```python
from build123d import *

# Parameters (mm, degrees)
EXTRUDE1_DEPTH = 5


with BuildPart() as part:
    # Sketch1 → Extrude1 (new body)
    with BuildSketch(Plane.XY):
        with BuildLine():
            Line((9.079809995, -4.626394269), (93.079809995, -47.426532026))
            ThreePointArc((93.079809995, -47.426532026), (101.052803287, -54.796691216), (104, -65.24666251))
            Line((104, -65.24666251), (104, -67))
            ThreePointArc((104, -67), (104.878679656, -69.121320344), (107, -70))
            Line((107, -70), (118.700463999, -70))
            ThreePointArc((118.700463999, -70), (120.442572866, -69.442346555), (121.537019726, -67.976704463))
            Line((121.537019726, -67.976704463), (140.410371512, -13.164510908))
            ThreePointArc((140.410371512, -13.164510908), (141.225712031, -9.954099936), (141.5, -6.653147818))
            Line((141.5, -6.653147818), (141.5, 17))
            ThreePointArc((141.5, 17), (140.621320344, 19.121320344), (138.5, 20))
            Line((138.5, 20), (122.5, 20))
            ThreePointArc((122.5, 20), (120.378679656, 19.121320344), (119.5, 17))
            Line((119.5, 17), (119.5, 16.5))
            ThreePointArc((119.5, 16.5), (95.5, -7.5), (71.5, 16.5))
            Line((71.5, 16.5), (71.5, 17))
            ThreePointArc((71.5, 17), (70.621320344, 19.121320344), (68.5, 20))
            Line((68.5, 20), (65, 20))
            ThreePointArc((65, 20), (62.878679656, 20.878679656), (62, 23))
            Line((62, 23), (62, 37))
            ThreePointArc((62, 37), (61.121320344, 39.121320344), (59, 40))
            Line((59, 40), (33.68653561, 40))
            ThreePointArc((33.68653561, 40), (31.795766306, 39.329161102), (30.750598067, 37.616660959))
            add(Edge.make_bspline(
                [(-38.750598067, 37.616660959), (-35.050414777, 20), (-4, 20), (27.050414777, 20), (30.750598067, 37.616660959)],
                knots=[3.261043467, 3.261043467, 3.261043467, 4.71238898, 4.71238898, 6.163734494, 6.163734494, 6.163734494], degree=2, weights=[1, 0.748053124, 1, 0.748053124, 1]))
            ThreePointArc((-38.750598067, 37.616660959), (-39.795766306, 39.329161102), (-41.68653561, 40))
            Line((-41.68653561, 40), (-54.5, 40))
            ThreePointArc((-54.5, 40), (-56.621320344, 39.121320344), (-57.5, 37))
            Line((-57.5, 37), (-57.5, 17.148970879))
            ThreePointArc((-57.5, 17.148970879), (-59.693566818, 5.888319313), (-65.953484912, -3.725599478))
            Line((-65.953484912, -3.725599478), (-87.272335061, -25.73069556))
            ThreePointArc((-87.272335061, -25.73069556), (-88.084372164, -27.372329), (-87.790703125, -29.180124095))
            Line((-87.790703125, -29.180124095), (-82.861971499, -38.853304561))
            ThreePointArc((-82.861971499, -38.853304561), (-81.11600291, -40.344502611), (-78.826980427, -40.164352635))
            Line((-78.826980427, -40.164352635), (-9.079809995, -4.626394269))
            ThreePointArc((-9.079809995, -4.626394269), (0, -2.446524753), (9.079809995, -4.626394269))
        make_face()
    extrude(amount=EXTRUDE1_DEPTH)


solid = part.part
```
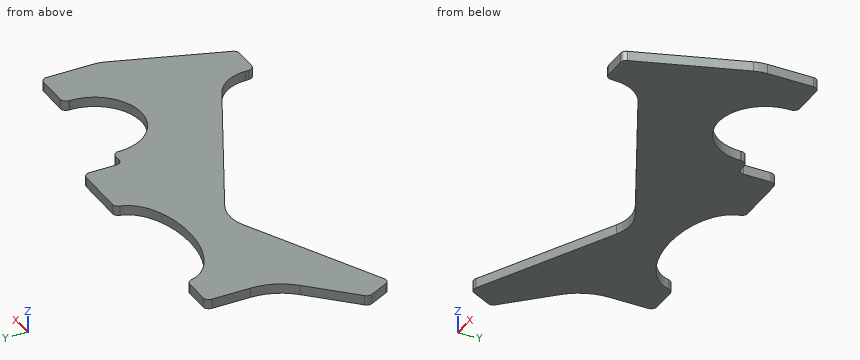
Here's how the part is built. I have some questions about the finished solid (model axes, mm). Coordinates: 2 decimals unless noted, no trailing zeros. Loops run counter-clockwise (first coordinate to the right, second up) from the corner with the lowest first, then second, coordinate; pieces in that order, holes last. Notation, with made-up numbers: (26.25, -3) - (61.25, -3) arc R16 ccw to (61.25, 9) - close; hole circle Ø7 at (-2, -32.5). An arc over 180 degrees is marked (long way). Return JSON: item names as keys, results as strings. Group by question number.
Item 1: Will these pins go through, and if not, where does the flat tip stop? P1, Ø3, axis at y = -17, z = 1.5, coming from the -X side; P2, Ø1.5, axis at y = 28.5, z = 3, coming from the -X side; P3, Ø1.9, axis at y = -66.5, z = 1.5, coming from the -X side.
Item 2: If we section it at B-B on x = 48.5: Write out the boundary of the cut face in (y, z).
Item 3: If we section it at A-A on x = 95.5: Write out the boundary of the cut face in (y, z).
Item 4: I need wall thicknesses on line 1 (X direction, y = -16.5, z = 0.6); line 2 (X direction, y = -20.5, z = 3.2); line 3 (Y direction, x = 66, z = 2.35). Which ranges of each line are inside material? Lowest first, please. Write a range as from..to.
Calculated:
{
 "1": {"P1": "stops at x = -80.27", "P2": "stops at x = -57.5", "P3": "stops at x = 104"},
 "2": {"outline": "(-24.71, 0) - (40, 0) - (40, 5) - (-24.71, 5) - close"},
 "3": {"outline": "(-48.88, 0) - (-7.5, 0) - (-7.5, 5) - (-48.88, 5) - close"},
 "4": {"line 1": "x = -78.33..-32.38, 32.38..139.26", "line 2": "x = -82.2..-40.23, 40.23..137.88", "line 3": "y = -33.63..20"}
}
